Could you check a few things on this model? Use its own coordinates, in mm. A direction names the side the tool comes from. Round coordinates to 2 decimals unless told otherwise and drop trailing zeros. Loops run counter-clockwise (first coordinate to the right, second up) from the corner with the lowest first, then second, coordinate; pieces in that order, holes last. Notation, with made-up numbers: (-36.5, 89.5) -> (-17.5, 89.5) arc R28 ccw to (-17.5, 109.5) -> close; hole circle Ø8 at (25, 15.25). An arc over 180 degrees is marked (long way). Write each question's results on one line, items separated by ' | '.
Autodesk Inventor part; units mm, degrees
ref_plane "YZ Plane" through (0, 0, 0) normal (1, 0, 0) x (0, 1, 0)
ref_plane "XZ Plane" through (0, 0, 0) normal (0, 1, 0) x (-1, 0, 0)
ref_plane "XY Plane" through (0, 0, 0) normal (0, 0, 1) x (1, 0, 0)
sketch "Sketch1" plane through (0, 0, 0) normal (0, 0, 1) x (1, 0, 0)
  line L0 (0, 0) -> (138.5, 0)
  line L1 (138.5, 0) -> (138.5, -28)
  line L2 (136.5, -30) -> (2, -30)
  line L3 (0, -28) -> (0, 0)
  line L4 (0, 0) -> (-3.5, 0)
  line L5 (-3.5, 0) -> (-3.5, -3)
  line L6 (-3.5, -3) -> (0, -3)
  line L7 (0, -3) -> (0, 0)
  line L8 (-3.5, 0) -> (-6.5, 0)
  line L9 (-6.5, 0) -> (-6.5, -10)
  line L10 (-6.5, -10) -> (-5.5, -10)
  line L11 (-3.5, -8) -> (-3.5, 0)
  line L12 (138.5, -3) -> (142, -3)
  line L13 (142, -3) -> (142, 0)
  line L14 (142, 0) -> (138.5, 0)
  line L15 (138.5, 0) -> (138.5, -3)
  line L16 (142, 0) -> (145, 0)
  line L17 (145, 0) -> (145, -10)
  line L18 (145, -10) -> (144, -10)
  line L19 (142, -8) -> (142, 0)
  arc A0 (-5.5, -10) -> (-3.5, -8) centre (-5.5, -8) ccw
  arc A1 (142, -8) -> (144, -10) centre (144, -8) ccw
  line L20 (5, -23) -> (55, -23)
  line L21 (55, -23) -> (55, -26)
  line L22 (55, -26) -> (5, -26)
  line L23 (5, -26) -> (5, -23)
  line L24 (83.5, -23) -> (133.5, -23)
  line L25 (133.5, -23) -> (133.5, -26)
  line L26 (133.5, -26) -> (83.5, -26)
  line L27 (83.5, -26) -> (83.5, -23)
  arc A2 (0, -28) -> (2, -30) centre (2, -28) ccw
  arc A3 (136.5, -30) -> (138.5, -28) centre (136.5, -28) ccw
  point P0 (138.5, -30)
  point P1 (0, -30)
  point P2 (-3.5, -10)
  point P3 (142, -10)
  dimension "d0" = 138.5
  dimension "d1" = 30
  dimension "d2" = 3.5
  dimension "d3" = 3
  dimension "d4" = 3
  dimension "d5" = 10
  dimension "d6" = 3.5
  dimension "d7" = 3
  dimension "d8" = 3
  dimension "d9" = 10
  dimension "d10" = 2
  dimension "d11" = 3
  dimension "d12" = 20
  dimension "d13" = 5
  dimension "d14" = 50
  dimension "d15" = 3
  dimension "d16" = 5
  dimension "d17" = 50
  dimension "d18" = 2
extrude "Extrusion1" add sketch "Sketch1" along normal blind 3
sketch "Sketch2" plane through (0, 0, 3) normal (0, 0, 1) x (1, 0, 0)
  line L0 (145, 0) -> (-6.5, 0)
  line L1 (10, 0) -> (128.5, 0)
  line L2 (128.5, 0) -> (128.5, 2)
  line L3 (108.5, -18) -> (30, -18)
  line L4 (10, 2) -> (10, 0)
  line L5 (5, -23) -> (55, -23)
  line L6 (0, -3) -> (0, -28)
  line L7 (138.5, -28) -> (138.5, -3)
  arc A0 (10, 2) -> (30, -18) centre (30, 2) ccw
  arc A1 (108.5, -18) -> (128.5, 2) centre (108.5, 2) ccw
  point P0 (0, 0)
  point P1 (128.3997, 0)
  point P2 (10.1003, 0)
  dimension "d21" = 5
  dimension "d22" = 10
  dimension "d23" = 10
  dimension "d24" = 20
extrude "Extrusion2" cut sketch "Sketch2" against normal blind 10 contours A1 L3 A0 L0
sketch "Sketch3" plane through (0, 0, 3) normal (0, 0, 1) x (1, 0, 0)
  arc A0 (10.1003, 0) -> (30, -18) centre (30, 2) ccw
  line L0 (10.1003, 0) -> (-6.5, 0)
  line L1 (-6.5, 0) -> (-6.5, -10)
  line L2 (-6.5, -10) -> (-5.5, -10)
  arc A1 (-5.5, -10) -> (-3.5, -8) centre (-5.5, -8) ccw
  line L3 (-3.5, -8) -> (-3.5, -3)
  line L4 (-3.5, -3) -> (0, -3)
  line L5 (0, -3) -> (0, -28)
  arc A2 (0, -28) -> (2, -30) centre (2, -28) ccw
  line L6 (2, -30) -> (136.5, -30)
  arc A3 (136.5, -30) -> (138.5, -28) centre (136.5, -28) ccw
  line L7 (138.5, -28) -> (138.5, -3)
  line L8 (138.5, -3) -> (142, -3)
  line L9 (142, -3) -> (142, -8)
  arc A4 (142, -8) -> (144, -10) centre (144, -8) ccw
  line L10 (144, -10) -> (145, -10)
  line L11 (145, -10) -> (145, 0)
  line L12 (145, 0) -> (128.3997, 0)
  arc A5 (108.5, -18) -> (128.3997, 0) centre (108.5, 2) ccw
  line L13 (108.5, -18) -> (30, -18)
  line L14 (83.5, -23) -> (133.5, -23)
  line L15 (133.5, -23) -> (133.5, -26)
  line L16 (133.5, -26) -> (83.5, -26)
  line L17 (83.5, -26) -> (83.5, -23)
  line L18 (5, -23) -> (55, -23)
  line L19 (55, -23) -> (55, -26)
  line L20 (55, -26) -> (5, -26)
  line L21 (5, -26) -> (5, -23)
  point P0 (0, 0)
equation "\"d15\" = d11"
equation "\"d16\" = d13"
equation "\"d17\" = d14"
properties part number "side"
1) I want a section at B-B, the plane z = 2.5. Write out the boundary of the cut face in (x, y).
Model answer:
outline: (-6.5, -10) -> (-5.5, -10) arc R2 ccw to (-3.5, -8) -> (-3.5, -3) -> (0, -3) -> (0, -28) arc R2 ccw to (2, -30) -> (136.5, -30) arc R2 ccw to (138.5, -28) -> (138.5, -3) -> (142, -3) -> (142, -8) arc R2 ccw to (144, -10) -> (145, -10) -> (145, 0) -> (128.4, 0) arc R20 cw to (108.5, -18) -> (30, -18) arc R20 cw to (10.1, 0) -> (-6.5, 0) -> close; hole (5, -26) -> (55, -26) -> (55, -23) -> (5, -23) -> close; hole (83.5, -26) -> (133.5, -26) -> (133.5, -23) -> (83.5, -23) -> close
2) I'm going to push flat-ended pins straight in: pin 1 (1.5 mm diameter, centred on y = -24.5, z = 2.5, fed in from +X); pin 2 (0.9 mm diameter, centred on y = -25, z = 1.5, fed in from -X). Where does each tip first touch, or does it pass through?
Model answer:
pin 1: stops at x = 138.5 | pin 2: stops at x = 0
3) If we mould it in two halves opening along X, with no side actions, what happens to faces 6 (the flat face through (-6.5, -5, 1)), 7 (the cylindrical face through (16.43, -12.69, 1.52)), 8 (the flat face through (68, -21, 3))? For each: released by +X, released by -X, zero draft, split by the parting line, or undercut.
Model answer:
face 6: released by -X | face 7: undercut | face 8: zero draft
4) I want a section at A-A, the plane x = 131.5. Write out the boundary of the cut face in (y, z), plus the area to 3 significant figures.
Model answer:
outline: (-30, 0) -> (-26, 0) -> (-26, 3) -> (-30, 3) -> close; (-23, 0) -> (0, 0) -> (0, 3) -> (-23, 3) -> close | area: 81.0 mm2
5) I want a section at D-D, the plane x = 82. Write out the boundary of the cut face in (y, z).
Model answer:
outline: (-30, 0) -> (-18, 0) -> (-18, 3) -> (-30, 3) -> close
6) I want a section at C-C, the plane y = -11.5. Write out the boundary of the cut face in (x, z), plus the area to 3 significant figures.
Model answer:
outline: (0, 0) -> (15.24, 0) -> (15.24, 3) -> (0, 3) -> close; (123.26, 0) -> (138.5, 0) -> (138.5, 3) -> (123.26, 3) -> close | area: 91.5 mm2
7) I need wall thicknesses on line 1 (X direction, y = -25, z = 1.3); line 2 (Y direction, x = 95, z = 0.75); line 3 (X direction, y = -11, z = 0.5). Which ranges of each line are inside material? Lowest first, please.
Model answer:
line 1: x = 0 to 5, 55 to 83.5, 133.5 to 138.5 | line 2: y = -30 to -26, -23 to -18 | line 3: x = 0 to 14.8, 123.7 to 138.5
8) For faces 1 (the flat face through (70, -18, 2)), 2 (the flat face through (2, 0, 1)), 3 (the flat face through (133.5, -24, 1)), 4 (the flat face through (0, -16, 1)), 5 (the flat face through (68, -21, 0)), which set-ups out of +Z, -Z, +X, -X, +Y, -Y let a thin tool reach every point of the face, with its end or its side?
Model answer:
face 1: +Z, -Z, +Y | face 2: +Z, -Z, +X, -X, +Y | face 3: +Z, -Z | face 4: +Z, -Z, -Y | face 5: -Z, +X, -X, +Y, -Y
